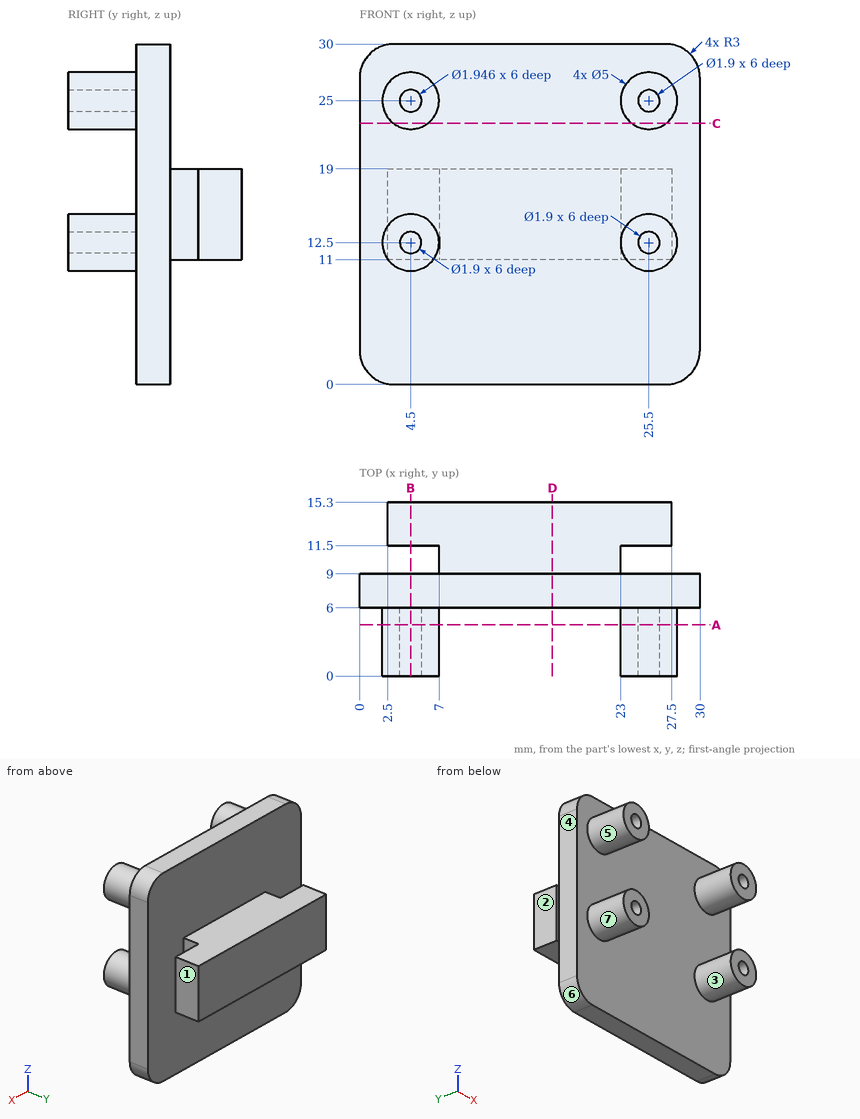
Design review of the part shown in the three views and the two pictorial views. Dimensions are in mm from the part's minimum x, y and z. A direction names the side the tool comes from. Round coordinates to 2 decimals unless told otherwise and drop trailing zeros. Loops run counter-clockwise (first coordinate to the right, second up) from the corner with the lowest first, then second, coordinate; pieces in that order, holes last.
1) The part is to be moulded in two halves that separate along Z. For the marked faces 4, 5, 6 and 7, say which applies: pulls with the +Z half, pulls with the -Z half, needs draft (parallel to the pull), parting line crosses it, or undercut.
Values follow:
face 4: needs draft
face 5: undercut
face 6: pulls with the -Z half
face 7: undercut
2) Clearance check with flat-ended pins moving along their axes: P1, Ø0.8, axis at y = 10.5, z = 15, coming from the -X side; P2, Ø1, axis at x = 19, z = 20.5, coming from the -Y side; P3, Ø1.9, axis at y = 13.5, z = 13.5, coming from the -X side; P4, Ø5, axis at x = 25.5, z = 14, coming from the -Y side. State where each tip first meets the part, or that it passes through.
Values follow:
P1: stops at x = 7
P2: stops at y = 6
P3: stops at x = 2.5
P4: stops at y = 0
3) Consider section C-C on z = 23. State the section outline as (x, y) points, then the cut area to 3 significant figures.
Values follow:
outline: (0, 6) - (3, 6) - (3, 0) - (6, 0) - (6, 6) - (24, 6) - (24, 0) - (27, 0) - (27, 6) - (30, 6) - (30, 9) - (0, 9) - close
area: 126 mm2
4) Wall thickness on line 1 along X through (y, z) = (2.8, 12.5); line 2 along X through (y, z) = (4.75, 25); line 3 along Y through (x, z) = (4, 16): over which ranges is each line inside the solid? List them lowest first.
Values follow:
line 1: x = 2 to 3.55, 5.45 to 7, 23 to 24.55, 26.45 to 28
line 2: x = 2 to 3.53, 5.47 to 7, 23 to 24.55, 26.45 to 28
line 3: y = 6 to 9, 11.5 to 15.3
5) Tool access review of the marked faces 1, 2 and 3: name each direction out of +Z, -Z, +X, -X, +Y, -Y from which nothing blocks a thin tool from reaching the whole face with its end or side.
Values follow:
face 1: +Z, -Z, +X, +Y
face 2: +Z, -Z, -X, +Y
face 3: -Y
6) Consider section A-A on y = 4.5. State the section outline as (x, z) points.
Values follow:
outline: circle Ø5 at (4.5, 12.5); circle Ø5 at (4.5, 25); circle Ø5 at (25.5, 12.5); circle Ø5 at (25.5, 25); hole circle Ø1.95 at (4.5, 25); hole circle Ø1.9 at (4.5, 12.5); hole circle Ø1.9 at (25.5, 12.5); hole circle Ø1.9 at (25.5, 25)
7) Consider section D-D on x = 17. State the section outline as (y, z) points, then the cut area to 3 significant figures.
Values follow:
outline: (6, 0) - (9, 0) - (9, 11) - (15.3, 11) - (15.3, 19) - (9, 19) - (9, 30) - (6, 30) - close
area: 140 mm2
8) Consider section B-B on x = 4.5. State the section outline as (y, z) points.
Values follow:
outline: (0, 10) - (6, 10) - (6, 0) - (9, 0) - (9, 30) - (6, 30) - (6, 27.5) - (0, 27.5) - (0, 25.97) - (6, 25.97) - (6, 24.03) - (0, 24.03) - (0, 22.5) - (6, 22.5) - (6, 15) - (0, 15) - (0, 13.45) - (6, 13.45) - (6, 11.55) - (0, 11.55) - close; (11.5, 11) - (15.3, 11) - (15.3, 19) - (11.5, 19) - close
